Model file for the job. Use its own axes, mm. Round coordinates to 2 decimals unless told otherwise and drop trailing zeros. Loops run counter-clockwise (first coordinate to the right, second up) from the corner with the lowest first, then second, coordinate; pieces in that order, holes last. Notation, with made-up numbers: (3.25, 62) -> (39.25, 62) arc R4 cw to (39.25, 69) -> close; hole circle Ø8 at (37.25, 77). An arc over 180 degrees is marked (long way). Use a Markdown table: item, result.
from build123d import *

# Parameters (mm, degrees)
F0_R     = 0.4
F1_DEPTH = 1
F2_R     = 0.3
F3_DEPTH = 0.55


with BuildPart() as f1:
    # F0 (on Top) → F1 (new body)
    with BuildSketch(Plane.XY):
        with BuildLine():
            Line((-9.5, -5), (9.5, -5))
            ThreePointArc((9.5, -5), (13.418354, 0), (9.5, 5))
            Line((9.5, 5), (-9.5, 5))
            ThreePointArc((-9.5, 5), (-13.44077, 0), (-9.5, -5))
        make_face()
        Circle(F0_R, mode=Mode.SUBTRACT)
    extrude(amount=F1_DEPTH)

    # F2 (on face) → F3 (join)
    with BuildSketch(Plane.XY.offset(1)):
        with BuildLine():
            Line((9.5, 5), (-9.5, 5))
            ThreePointArc((-9.5, 5), (-13.44077, 0), (-9.5, -5))
            Line((-9.5, -5), (9.5, -5))
            ThreePointArc((9.5, -5), (13.418354, 0), (9.5, 5))
        make_face()
        Circle(F2_R, mode=Mode.SUBTRACT)
    extrude(amount=F3_DEPTH)


solid = f1.part
Q1. Band-saw the part on C-C, the plane z = 0.5. Give the cut face in (x, y).
Results list:
| item | result |
|---|---|
| outline | (-9.5, -5) -> (9.5, -5) arc R5.15 ccw to (9.5, 5) -> (-9.5, 5) arc R5.14 ccw to start; hole circle Ø0.8 at (0, 0) |
Q2. Band-saw the part on B-B, the plane x = 0. Give the cut face in (y, z), plus the area to 3 significant figures.
Results list:
| item | result |
|---|---|
| outline | (-5, 0) -> (-0.4, 0) -> (-0.4, 1) -> (-0.3, 1) -> (-0.3, 1.55) -> (-5, 1.55) -> close; (0.3, 1) -> (0.4, 1) -> (0.4, 0) -> (5, 0) -> (5, 1.55) -> (0.3, 1.55) -> close |
| area | 14.4 mm² |
Q3. Band-saw the part on D-D, the plane y = 2.5. Give the cut face in (x, z).
Results list:
| item | result |
|---|---|
| outline | (-12.79, 0) -> (12.77, 0) -> (12.77, 1.55) -> (-12.79, 1.55) -> close |
Q4. Band-saw the part on A-A, the plane y = 0. Give the cut face in (x, z).
Results list:
| item | result |
|---|---|
| outline | (-13.44, 0) -> (-0.4, 0) -> (-0.4, 1) -> (-0.3, 1) -> (-0.3, 1.55) -> (-13.44, 1.55) -> close; (0.3, 1) -> (0.4, 1) -> (0.4, 0) -> (13.42, 0) -> (13.42, 1.55) -> (0.3, 1.55) -> close |
Q5. Drill centre lines: L1, parallel to Y at x = 0, z = 0.75; L2, parallel to Y at x = 0, z = 1.15; L3, parallel to Y at x = 12.5, z = 1.3. Where is each one in solid material? Low to high. Write a range as from..to.
Results list:
| item | result |
|---|---|
| L1 | y = -5..-0.4, 0.4..5 |
| L2 | y = -5..-0.3, 0.3..5 |
| L3 | y = -2.94..2.94 |
